Build history of the part. All positions in model axes, mm. A direction names the side the tool comes from. Coordinates: 2 decimals unless noted, no trailing zeros. Write each loop counter-clockwise with the first axis right and the second up, starting at its lowest first coordinate (ties: lowest second). Pieces come first, ordered by that corner, then holes.
```python
from build123d import *

# Parameters (mm, degrees)
EXTRUDE_1_DEPTH          = 30
CUT_EXTRUDE_1_DEPTH      = 74.890488337
CUT_EXTRUDE_1_DEPTH_BACK = 74.890488337
SKETCH_2_R               = 10
SKETCH_4_W               = 10
SKETCH_4_H               = 10
CUT_EXTRUDE_2_DEPTH      = 71.426335574


with BuildPart() as part:
    # 스케치1 → 보스-돌출1 (new body)
    with BuildSketch(Plane(origin=(0, 0, 0), x_dir=(1, 0, 0), z_dir=(0, 1, 0))):
        Polygon((-30.496316142, 3.867716008), (-30.496316142, 13.866104182), (-60.496316142, 13.866104182), (-60.496316142, 23.867716008), (-30.496316142, 23.867716008), (-30.496316142, 33.867716008), (9.503683858, 33.867716008), (9.503683858, 25.867716008), (-22.496316142, 25.867716008), (-22.496316142, 11.867716008), (9.503683858, 11.867716008), (9.503683858, 3.867716008), align=None)
    extrude(amount=EXTRUDE_1_DEPTH)

    # 스케치2 → 컷-돌출1 (cut, two sides: drawn at the far end of the back side and taken through both)
    with BuildSketch(Plane.XY.offset(-3.867716008).offset(-CUT_EXTRUDE_1_DEPTH_BACK)):
        with Locations((-10.496316142, 15)):
            Circle(SKETCH_2_R)
    extrude(amount=CUT_EXTRUDE_1_DEPTH + CUT_EXTRUDE_1_DEPTH_BACK, mode=Mode.SUBTRACT)

    # 스케치4 → 컷-돌출2 (cut, through all)
    with BuildSketch(Plane.XY.offset(-13.866104182)):
        with Locations((-45.496316142, 15)):
            Rectangle(SKETCH_4_W, SKETCH_4_H)
    extrude(amount=-CUT_EXTRUDE_2_DEPTH, mode=Mode.SUBTRACT)


solid = part.part
```
1. Saw through at C-C on x = -15. List the corners of the cut face in (y, z).
Computed values:
outline: (0, -33.87) - (6.07, -33.87) - (6.07, -25.87) - (0, -25.87) - close; (0, -11.87) - (6.07, -11.87) - (6.07, -3.87) - (0, -3.87) - close; (23.93, -33.87) - (30, -33.87) - (30, -25.87) - (23.93, -25.87) - close; (23.93, -11.87) - (30, -11.87) - (30, -3.87) - (23.93, -3.87) - close
2. Saw through at B-B on z = -17.5. List the corners of the cut face in (x, y), plus the area to 3 significant figures.
Computed values:
outline: (-60.5, 0) - (-22.5, 0) - (-22.5, 30) - (-60.5, 30) - close; hole (-50.5, 10) - (-40.5, 10) - (-40.5, 20) - (-50.5, 20) - close
area: 1,040 mm2
3. Mould opens along Z. For faces 1 (the face through (-52, 15, -13.866)), 2 (the face through (1, 15, -25.868)), 3 (the face through (-50.496, 15, -19)), 4 (the face through (-39, 15, -23.868)) say: +Z half, -Z half, draft (parallel to the pull), parting line (faces both ways), or undercut.
Computed values:
face 1: +Z half
face 2: undercut
face 3: draft
face 4: -Z half
4. 3-axis set-ups, long thin cutter, end or side, ignore diameter. For faces 5 (the face through (-46, 20, -19)), 6 (the face through (-30.496, 15, -29)), 7 (the face through (-22.496, 15, -19)), 8 (the face through (9.504, 15, -30)), 9 (the face through (-30.496, 15, -9)): which of +Z, -Z, +X, -X, +Y, -Y reach the whole face in a straight line?
Computed values:
face 5: +Z, -Z
face 6: -Z, -X, +Y, -Y
face 7: +X, +Y, -Y
face 8: +Z, -Z, +X, +Y, -Y
face 9: +Z, -X, +Y, -Y
5. Probe line 1 along Z through (x, y) = (-0.5, 12.25); line 2 along X through (y, z) = (18, -14); line 3 along X through (y, z) = (15, -5.5). List the from-to ranges inside material, lowest first.
Computed values:
line 1: z = -33.87 to -25.87, -11.87 to -3.87
line 2: x = -60.5 to -50.5, -40.5 to -22.5
line 3: x = -30.5 to -20.5, -0.5 to 9.5
6. Saw through at D-D on y = 28. List the corners of the cut face in (x, z).
Computed values:
outline: (-60.5, -23.87) - (-30.5, -23.87) - (-30.5, -33.87) - (9.5, -33.87) - (9.5, -25.87) - (-22.5, -25.87) - (-22.5, -11.87) - (9.5, -11.87) - (9.5, -3.87) - (-30.5, -3.87) - (-30.5, -13.87) - (-60.5, -13.87) - close
7. Flat gauge pins, fed straight in: pin 1 (11 mm diameter, centred on y = 20, z = -19, fed in from +X); pin 2 (8 mm diameter, centred on x = -44.5, y = 19, fed in from +Z); pin 3 (6 mm diameter, centred on y = 20, z = -9.5, fed in from -X). Where does each tip first touch, or does it go through?
Computed values:
pin 1: stops at x = -22.5
pin 2: stops at z = -13.87
pin 3: stops at x = -30.5
8. Saw through at A-A on y = 15. List the corners of the cut face in (x, z), plus the area to 3 significant figures.
Computed values:
outline: (-60.5, -23.87) - (-50.5, -23.87) - (-50.5, -13.87) - (-60.5, -13.87) - close; (-40.5, -23.87) - (-30.5, -23.87) - (-30.5, -33.87) - (-20.5, -33.87) - (-20.5, -25.87) - (-22.5, -25.87) - (-22.5, -11.87) - (-20.5, -11.87) - (-20.5, -3.87) - (-30.5, -3.87) - (-30.5, -13.87) - (-40.5, -13.87) - close; (-0.5, -33.87) - (9.5, -33.87) - (9.5, -25.87) - (-0.5, -25.87) - close; (-0.5, -11.87) - (9.5, -11.87) - (9.5, -3.87) - (-0.5, -3.87) - close
area: 632 mm2
